Model file for the job. Use its own axes, mm. Round coordinates to 2 decimals unless told otherwise and drop trailing zeros. Order: outer loops, then holes, each group sorted by start corner. A loop starts at its lowest first (then second) coordinate and runs counter-clockwise, first axis right, second up. Notation, with made-up numbers: (4.5, -38.75) - (17.5, -38.75) arc R16 ccw to (17.5, -14.75) - close; hole circle Ø6 at (30, 27.25). An arc over 180 degrees is marked (long way). Write item = value, one per line.
```python
from build123d import *

# Parameters (mm, degrees)
SKETCH1_R           = 10
BOSS_EXTRUDE1_DEPTH = 10
SKETCH2_R           = 10
BOSS_EXTRUDE2_DEPTH = 60
SWEEP1_START        = -1000
SWEEP1_OUTLINE_R    = 10
SWEEP1_DEPTH        = 940
SWEEP1_START_2      = -230.0000001
SWEEP1_2_OUTLINE_R  = 10
SWEEP1_2_DEPTH      = 240.0000001
SWEEP1_3_OUTLINE_R  = 10
SWEEP1_3_ANGLE      = 90


with BuildPart() as part:
    # Sketch1 → Boss-Extrude1 (new body)
    with BuildSketch(Plane(origin=(0, 0, 0), x_dir=(1, 0, 0), z_dir=(0, 1, 0))):
        with BuildLine():
            ThreePointArc((14.831374996, 67.242836537), (0, 80), (-14.831374996, 67.242836537))
            Line((-14.831374996, 67.242836537), (-23.88215206, 7.392077718))
            Line((-23.88215206, 7.392077718), (-25, 0))
            ThreePointArc((-25, 0), (0, -25), (25, 0))
            Line((25, 0), (23.88215206, 7.392077718))
            Line((23.88215206, 7.392077718), (14.831374996, 67.242836537))
        make_face()
        with Locations(Location((0, 0, 0), (0, 0, 270))):
            Circle(SKETCH1_R, mode=Mode.SUBTRACT)
    extrude(amount=BOSS_EXTRUDE1_DEPTH)

    # Sketch2 → Boss-Extrude2 (add)
    with BuildSketch(Plane(origin=(0, 10, 0), x_dir=(1, 0, 0), z_dir=(0, 1, 0))):
        with Locations(Location((0, 64.677844525, 0), (0, 0, 270))):
            Circle(SKETCH2_R)
    extrude(amount=BOSS_EXTRUDE2_DEPTH)

    # Sweep1 2 outline → Sweep1 2 (add)
    with BuildSketch(Plane(origin=(0, 0, 0), x_dir=(1, 0, 0), z_dir=(0, 1, 0)).offset(SWEEP1_START_2)):
        Circle(SWEEP1_2_OUTLINE_R)
    extrude(amount=SWEEP1_2_DEPTH)



with BuildPart() as body_2:
    # Sweep1: read off the stored shape, not the designer's step
    # Sweep1 outline → Sweep1 (new body)
    with BuildSketch(Plane.XY.offset(SWEEP1_START)):
        with Locations((0, -290)):
            Circle(SWEEP1_OUTLINE_R)
    extrude(amount=SWEEP1_DEPTH)


with BuildPart() as part_1:
    add(part.part)

    add(body_2.part)  # Sweep1 3 merges body 2
    # Sweep1 3 outline → Sweep1 3 (revolve)
    with BuildSketch(Plane(origin=(0, -230, -60), x_dir=(0, 0, 1), z_dir=(0, 1, 0))):
        with Locations((60, 0)):
            Circle(SWEEP1_3_OUTLINE_R)
    revolve(axis=Axis((0, -230, -60), (1, 0, 0)), revolution_arc=SWEEP1_3_ANGLE)


solid = part_1.part
```
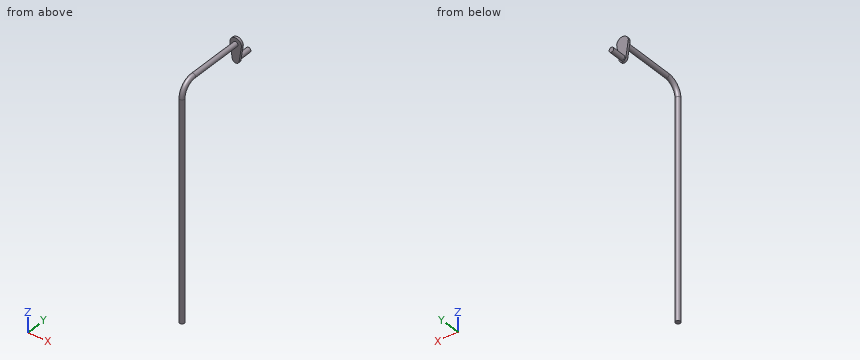
1) Cut at B-B (z = -691). Write the cut outline in (x, y).
Conclusion:
outline = circle Ø20 at (0, -290)
2) Flat gauge pins, fed straight in: pin 1 Ø6 at (x, y) = (2, -226) entering from +Z; pin 2 Ø12 at (x, z) = (1.5, -600) entering from +Y; pin 3 Ø4 at (x, z) = (7, -449) entering from -Y. Where does each tip first touch, or does it go through?
Conclusion:
pin_1 = 10
pin_2 = -280
pin_3 = -298.66
3) Cut at C-C (y = 22.5). Write the cut outline in (x, z).
Conclusion:
outline = circle Ø20 at (0, -64.68)
4) Cut at A-A (x = 0). Write the cut outline in (y, z), and give its area (3 significant figures).
Conclusion:
outline = (-300, -1000) - (-280, -1000) - (-280, -60) arc R50 cw to (-230, -10) - (0, -10) - (0, -80) - (10, -80) - (10, -74.68) - (70, -74.68) - (70, -54.68) - (10, -54.68) - (10, 25) - (0, 25) - (0, 10) - (-230, 10) arc R70 ccw to (-300, -60) - close
area = 27,500 mm^2
5) Wall check: line 1 along Z through (x, y) = (0, -177.5); line 2 along Y through (x, z) = (-7.5, -823); line 3 along Z through (x, y) = (-1, -211.5). Give the ranges that are in metal, low to high.
Conclusion:
line_1 = -10 to 10
line_2 = -296.61 to -283.39
line_3 = -9.95 to 9.95
